from build123d import *

# Parameters (mm, degrees)
BOSS_EXTRUDE1_DEPTH = 5
SKETCH8_W           = 20.178262132
SKETCH8_H           = 15
BOSS_EXTRUDE2_DEPTH = 5
SHELL4_DEPTH        = 4
SHELL4_START        = -5
SHELL4_2_OUTLINE_W  = 18.178262132
SHELL4_2_OUTLINE_H  = 13
SHELL4_2_DEPTH      = 5
SKETCH9_R           = 2.45
CUT_EXTRUDE3_DEPTH  = 56.455798629
SKETCH10_R          = 2.25
CUT_EXTRUDE4_DEPTH  = 10


# Read off the part's stored shape, not the designer's step: Shell4
with BuildPart() as part:
    # Sketch2 → Boss-Extrude1 (new body)
    with BuildSketch(Plane(origin=(0, 0, 0), x_dir=(1, 0, 0), z_dir=(0, 1, 0))):
        with BuildLine():
            Line((-39.115, 0.880622479), (-39.115, 10))
            Line((-39.115, 10), (39.115, 10))
            Line((39.115, 10), (39.115, 0.880622479))
            Line((39.115, 0.880622479), (39.115, -4.119377521))
            Line((39.115, -4.119377521), (14.608241959, -4.119377521))
            ThreePointArc((14.608241959, -4.119377521), (11.072708053, -5.583843615), (9.608241959, -9.119377521))
            Line((9.608241959, -9.119377521), (9.608241959, -24.119377521))
            Line((9.608241959, -24.119377521), (-10.570020173, -24.119377521))
            Line((-10.570020173, -24.119377521), (-10.570020173, -9.119377521))
            ThreePointArc((-10.570020173, -9.119377521), (-12.034486267, -5.583843615), (-15.570020173, -4.119377521))
            Line((-15.570020173, -4.119377521), (-39.115, -4.119377521))
            Line((-39.115, -4.119377521), (-39.115, 0.880622479))
        make_face()
    extrude(amount=BOSS_EXTRUDE1_DEPTH)

    # Sketch8 → Boss-Extrude2 (add)
    with BuildSketch(Plane.XZ):
        with Locations((-0.480889107, 16.619377521)):
            Rectangle(SKETCH8_W, SKETCH8_H)
    extrude(amount=BOSS_EXTRUDE2_DEPTH)

    # Shell4 outline → Shell4 (cut)
    with BuildSketch(Plane(origin=(0, 0, 0), x_dir=(1, 0, 0), z_dir=(0, 1, 0))):
        with BuildLine():
            Line((38.115, 9), (-38.115, 9))
            Line((-38.115, 9), (-38.115, -3.119377521))
            Line((-38.115, -3.119377521), (-15.570020173, -3.119377521))
            ThreePointArc((-15.570020173, -3.119377521), (-11.327379486, -4.876736834), (-9.570020173, -9.119377521))
            Line((-9.570020173, -9.119377521), (-9.570020173, -23.119377521))
            Line((-9.570020173, -23.119377521), (8.608241959, -23.119377521))
            Line((8.608241959, -23.119377521), (8.608241959, -9.119377521))
            ThreePointArc((8.608241959, -9.119377521), (10.365601272, -4.876736834), (14.608241959, -3.119377521))
            Line((14.608241959, -3.119377521), (38.115, -3.119377521))
            Line((38.115, -3.119377521), (38.115, 9))
        make_face()
    extrude(amount=SHELL4_DEPTH, mode=Mode.SUBTRACT)

    # Shell4 2 outline → Shell4 2 (cut)
    with BuildSketch(Plane(origin=(0, 0, 0), x_dir=(1, 0, 0), z_dir=(0, 1, 0)).offset(SHELL4_START)):
        with Locations((-0.480889107, -16.619377521)):
            Rectangle(SHELL4_2_OUTLINE_W, SHELL4_2_OUTLINE_H)
    extrude(amount=SHELL4_2_DEPTH, mode=Mode.SUBTRACT)

    # Sketch9 → Cut-Extrude3 (cut, through all)
    with BuildSketch(Plane.ZY.offset(10.570020173)):
        with Locations((16.119377521, 0)):
            Circle(SKETCH9_R)
    extrude(amount=-CUT_EXTRUDE3_DEPTH, mode=Mode.SUBTRACT)

    # Sketch10 → Cut-Extrude4 (cut)
    with BuildSketch(Plane(origin=(0, 5, 0), x_dir=(1, 0, 0), z_dir=(0, 1, 0))):
        with Locations(Location((-32.115, 5, 0), (0, 0, 270))):
            Circle(SKETCH10_R)
        with Locations(Location((-22.775, 5, 0), (0, 0, 270))):
            Circle(SKETCH10_R)
        with Locations(Location((32.115, 0, 0), (0, 0, 270))):
            Circle(SKETCH10_R)
        with Locations(Location((22.775, 0, 0), (0, 0, 270))):
            Circle(SKETCH10_R)
    extrude(amount=-CUT_EXTRUDE4_DEPTH, mode=Mode.SUBTRACT)


solid = part.part
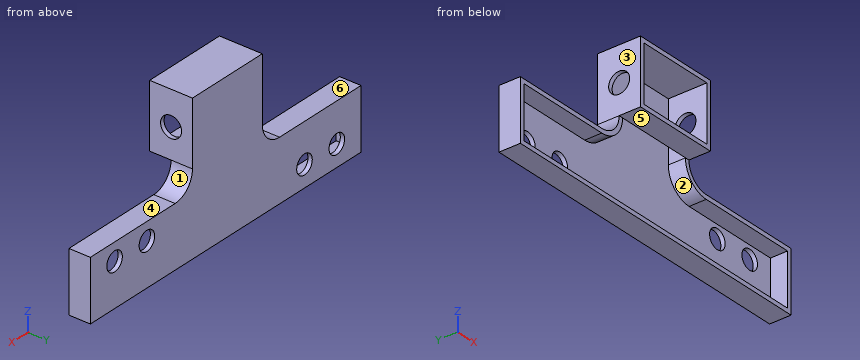
Could you check a few things on this model? Use its own coordinates, in mm. Face numbers are marked on the shaded views. A direction names the side the tool comes from. Give positions to 0.01 mm unless a question says otherwise; leave off trailing zeros. Order: outer loops, then holes, each group sorted by start corner. A loop starts at its lowest first (then second) coordinate and runs counter-clockwise, first axis right, second up. Notation, with made-up numbers: (-20.5, 77.5) -> (-10.5, 77.5) arc R19 ccw to (-10.5, 105.5) -> close; hole circle Ø2 at (24, 61.5). An arc over 180 degrees is marked (long way). Answer in a Markdown table with one row per item. Add a question column.
Item 1: Imagine slicing it at B-B (y = -3.5). List the corners of the cut face in (x, z) for me.
Item 2: Imagine slicing it at C-C (x = -8.5). List the corners of the cut face in (y, z) for me, and give its area (3 significant figures).
Item 3: Imagine slicing it at D-D (x = -26.5). List the corners of the cut face in (y, z) for me, and give its area (3 significant figures).
Item 4: We'd pull the mould along X, two halves only. Please class the marked faces 1, 2 and 3: pulls with the +X half, pulls with the -X half, needs draft (parallel to the pull), parting line crosses it, or undercut.
Item 5: I'm going to push flat-ended pins straight in: P1, Ø3, axis at y = 1, z = 18.5, coming from the +X side; P2, Ø5, axis at x = 28.5, z = -1, coming from the -Y side; P3, Ø1.5, axis at y = -1, z = -6, coming from the +X side (3 decimals); P4, Ø16, axis at x = -19, z = 12, coming from the -Y side. Where does each tip first touch, or does it pass through?
Item 6: Please list where these lines run through material, in increasing order: probe 1 along X at (y, z) = (4.3, -5) (3 decimals); probe 2 along Z at (x, y) = (-2.5, -1); probe 3 along X at (y, z) = (3.5, 21).
Item 7: For the marked faces 4, 5 and 6, which set-ups out of +Z, -Z, +X, -X, +Y, -Y let a thin tool reach every point of the face, with its end or its side?
Item 8: Imagine slicing it at A-A (z = 0). List the corners of the cut face in (x, y) for me (3 decimals), and give its area (3 significant figures).
Result:
| question | item | result |
|---|---|---|
| 1 | outline | (-10.57, 9.12) -> (9.61, 9.12) -> (9.61, 24.12) -> (-10.57, 24.12) -> close; hole (-9.57, 10.12) -> (8.61, 10.12) -> (8.61, 23.12) -> (-9.57, 23.12) -> close |
| 2 | outline | (-5, 9.12) -> (0, 9.12) -> (0, 10.12) -> (-5, 10.12) -> close; (-5, 23.12) -> (4, 23.12) -> (4, -9) -> (0, -9) -> (0, -10) -> (5, -10) -> (5, 24.12) -> (-5, 24.12) -> close |
| 2 | area | 52.1 mm2 |
| 3 | outline | (0, -10) -> (5, -10) -> (5, 4.12) -> (0, 4.12) -> (0, 3.12) -> (4, 3.12) -> (4, -9) -> (0, -9) -> close |
| 3 | area | 22.1 mm2 |
| 4 | face 1 | pulls with the +X half |
| 4 | face 2 | undercut |
| 4 | face 3 | pulls with the -X half |
| 5 | P1 | x = 9.61 |
| 5 | P2 | y = 4 |
| 5 | P3 | through |
| 5 | P4 | y = 0 |
| 6 | probe 1 | -39.115 to -34.365, -29.865 to -25.025, -20.525 to 39.115 |
| 6 | probe 2 | 9.12 to 10.12, 23.12 to 24.12 |
| 6 | probe 3 | -10.57 to -9.57, 8.61 to 9.61 |
| 7 | face 4 | +Z, +X, +Y, -Y |
| 7 | face 5 | -Z, +X, -X, -Y |
| 7 | face 6 | +Z, -X, +Y, -Y |
| 8 | outline | (-39.115, 0) -> (-38.115, 0) -> (-38.115, 4) -> (20.525, 4) -> (20.525, 5) -> (-39.115, 5) -> close; (25.025, 4) -> (29.865, 4) -> (29.865, 5) -> (25.025, 5) -> close; (34.365, 4) -> (38.115, 4) -> (38.115, 0) -> (39.115, 0) -> (39.115, 5) -> (34.365, 5) -> close |
| 8 | area | 77.2 mm2 |
